Can you work these out from the model? Positions are in its coordinate system, mm. Face numbers are marked on the shaded views. Coordinates: 2 decimals unless noted, no trailing zeros. Write each loop counter-clockwise with the first axis right and the second up, starting at its lowest first coordinate (ties: lowest second). Pieces come first, ordered by that corner, then holes. Notation, with made-up numbers: (-38.75, 61) - (0.25, 61) arc R28 cw to (0.25, 91) - close; hole circle Ø7 at (-40, 70). An arc over 180 degrees is marked (long way). Write each question's results on one line, items separated by ' | '. Start each with the question number.
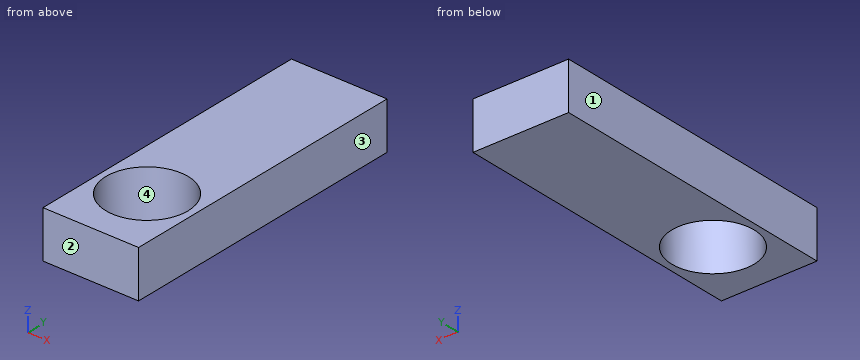
```python
from build123d import *

# Parameters (mm, degrees)
F0_W     = 81.611588
F0_H     = 40.411144
F1_DEPTH = 254
F2_R     = 35.152573
F3_DEPTH = 254


with BuildPart() as f1:
    # F0 (on Front) → F1 (new body)
    with BuildSketch(Plane.XZ):
        with Locations((13.023123, 10.158926)):
            Rectangle(F0_W, F0_H)
    extrude(amount=F1_DEPTH)

    # F2 (on face) → F3 (cut)
    with BuildSketch(Plane.XY.offset(30.364498)):
        with Locations((12.749678, -196.172729)):
            Circle(F2_R)
    extrude(amount=-F3_DEPTH, mode=Mode.SUBTRACT)


solid = f1.part
```
Q1. If we section it at B-B (x = 3.5): Please give me the cut outline in (y, z), then the cut area to 3 significant figures.
Q2. I need wall thicknesses on line 1 along Y through (x, z) = (13, 9); line 2 along Y through (x, z) = (11, 8); line 3 along X through (y, z) = (-197.5, 1). Which ranges of each line are inside material? Lowest first, please. Write a range as from..to.
Q3. If we section it at A-A (y = -213): Please give me the cut outline in (x, z).
Q4. Thinking about a two-plate mould opening in X: for the marked faces 1, 2, 3 and 4, which applies, pulls with the +X half, pulls with the -X half, needs draft (parallel to the pull), parting line crosses it, or undercut?
Q5. If we section it at C-C (z = 1): Please give me the cut outline in (x, y), then the cut area to 3 significant figures.
Answer list:
1) outline: (-254, -10.05) - (-230.09, -10.05) - (-230.09, 30.36) - (-254, 30.36) - close; (-162.26, -10.05) - (0, -10.05) - (0, 30.36) - (-162.26, 30.36) - close | area: 7,520 mm2
2) line 1: y = -254..-231.32, -161.02..0 | line 2: y = -254..-231.28, -161.06..0 | line 3: x = -27.78..-22.38, 47.88..53.83
3) outline: (-27.78, -10.05) - (-18.11, -10.05) - (-18.11, 30.36) - (-27.78, 30.36) - close; (43.61, -10.05) - (53.83, -10.05) - (53.83, 30.36) - (43.61, 30.36) - close
4) face 1: pulls with the -X half | face 2: needs draft | face 3: pulls with the +X half | face 4: undercut
5) outline: (-27.78, -254) - (53.83, -254) - (53.83, 0) - (-27.78, 0) - close; hole circle Ø70.31 at (12.75, -196.17) | area: 16,800 mm2
